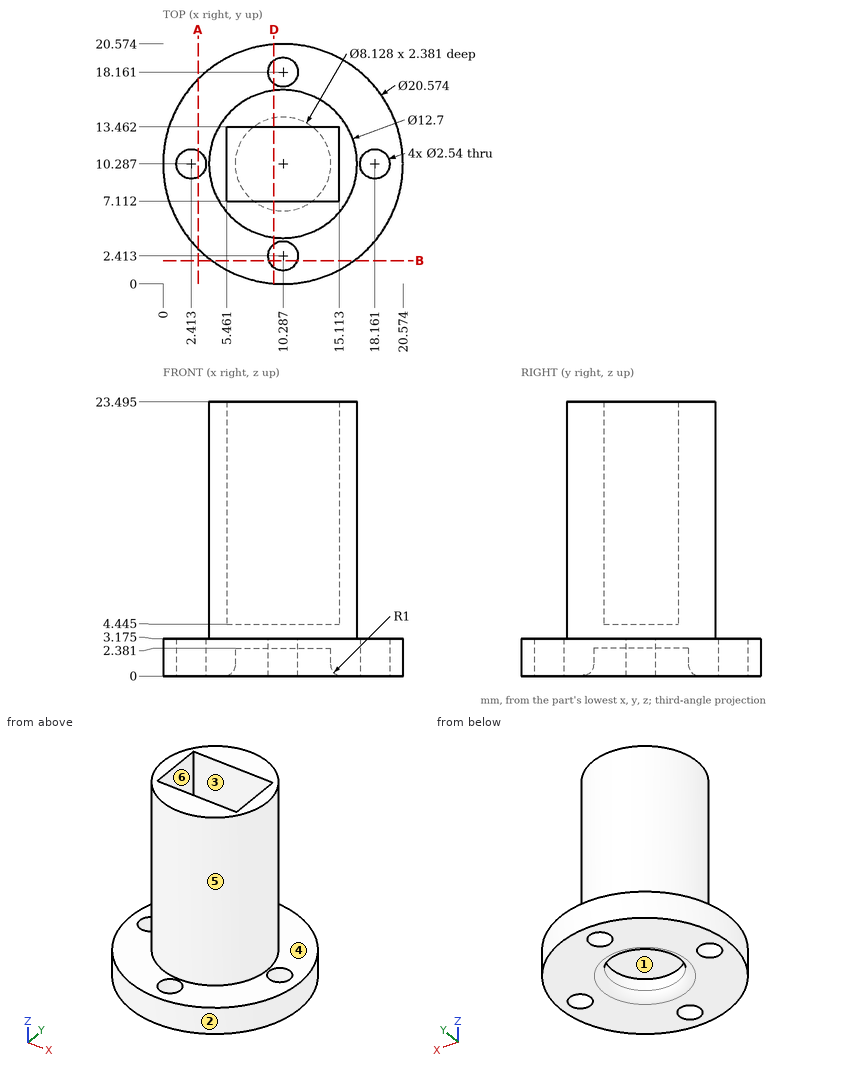
Job drawing, mm, ordinate dimensions from the low corner. One solid piece. A direction names the side the tool comes from. Give positions to 0.01 mm unless a question says otherwise; leave off trailing zeros. Order: outer loops, then holes, each group sorted by start corner. A loop starts at its lowest first (then second) coordinate and runs counter-clockwise, first axis right, second up. Notation, with made-up numbers: (20, 26) - (45, 26) arc R25 cw to (45, 56) - close; hole circle Ø11 at (-26, 19.5). An arc over 180 degrees is marked (long way). Answer in a Markdown table with one row per item.
1. Pull direction X, two halves, no side cores. Call the marked faces 4, 5 and 6: pulls with the +X half, pulls with the -X half, needs draft (parallel to the pull), parting line crosses it, or undercut.
Data:
| item | result |
|---|---|
| face 4 | needs draft |
| face 5 | parting line crosses it |
| face 6 | undercut |
2. Saw through at B-B, the plane y = 2. Give the cut face in (x, z) (1 decimal).
Data:
| item | result |
|---|---|
| outline | (4.2, 0) - (9.1, 0) - (9.1, 3.2) - (4.2, 3.2) - close; (11.5, 0) - (16.4, 0) - (16.4, 3.2) - (11.5, 3.2) - close |
3. Tool access for the marked faces 1, 2 and 3: list every direction of +Z, -Z, +X, -X, +Y, -Y with a clear straight run to the whole face (end or side of a thin tool).
Data:
| item | result |
|---|---|
| face 1 | -Z |
| face 2 | +Z, -Z |
| face 3 | +Z |
4. Saw through at A-A, the plane x = 3. Give the cut face in (y, z) (1 decimal).
Data:
| item | result |
|---|---|
| outline | (3, 0) - (9.2, 0) - (9.2, 3.2) - (3, 3.2) - close; (11.4, 0) - (17.5, 0) - (17.5, 3.2) - (11.4, 3.2) - close |
5. Saw through at D-D, the plane x = 9.5. Count the separate pieces of the cut face and the enclosed holes in it, plus the area to 3 significant figures.
Data:
| item | result |
|---|---|
| separate pieces | 3 |
| enclosed holes | 0 |
| area | 168 mm² |
6. Probe probe 1 along Y at (x, z) = (10.25, 5.25); probe 2 along X at (y, z) = (11.5, 10.5); probe 3 along Y at (x, z) = (5.5, 6.5) (1 decimal). List the from-to ranges inside material, lowest first. Write a range as [from, to].
Data:
| item | result |
|---|---|
| probe 1 | y = [3.94, 7.11], [13.46, 16.64] |
| probe 2 | x = [4.05, 5.46], [15.11, 16.52] |
| probe 3 | y = [6.1, 7.1], [13.5, 14.5] |
7. Flat gauge pins, fed straight in: pin 1 (3 mm diameter, centred on y = 6.5, z = 19.5, fed in from +X); pin 2 (7.5 mm diameter, centred on x = 12.5, z = 16, fed in from +Y); pin 3 (5 mm diameter, centred on x = 9.5, z = 15, fed in from -Y). Where does each tip first touch, or does it go through?
Data:
| item | result |
|---|---|
| pin 1 | stops at x = 16.21 |
| pin 2 | stops at y = 16.64 |
| pin 3 | stops at y = 3.94 |
